For this review, take the finished solid that the model builds, in its own axes (mm). A direction names the side the tool comes from. Round coordinates to 2 decimals unless told otherwise and drop trailing zeros. Write each loop counter-clockwise with the first axis right and the second up, starting at its lowest first coordinate (ties: lowest second). Pieces come first, ordered by that corner, then holes. Notation, with made-up numbers: (-24, 80) -> (18, 80) arc R27 cw to (18, 107) -> close; hole circle Ø4 at (-31, -36.75). An arc over 180 degrees is marked (long way). Answer as CSV lines item,"result". Start each with the question number.
Item 1: Take a section at C-C on x = -47. Give the boundary of the cut face in (y, z).
Item 2: Take a section at D-D on x = 3. Give the boundary of the cut face in (y, z), then the cut area to 3 significant figures.
Item 3: Machinability: for faces 4 (the flat face through (-14, -12, 4)), 5 (the flat face through (0, 0, 8)), which of the approach directions +Z, -Z, +X, -X, +Y, -Y give a long, thin tool a straight path to every point of the face, cutting with its end or side? Answer none if there is none.
Item 4: Mouldability with a two-part tool opening along Y and no side actions: class faces 1 (the cylindrical face through (24.4, -44.6, 2)), 2 (the cylindrical face through (-13.887, -10.648, 5.972)), 3 (the flat face through (-1, 1, 0)) as +Y half, -Y half, draft (parallel to the pull), parting line (faces both ways), or undercut.
Item 5: For pin 1 Ø1.5 at (y, z) = (-25.5, 1) entering from +X; pin 2 Ø10 at (x, y) = (-43.5, -30.5) entering from +Z; pin 3 Ø5 at (x, y) = (23.5, -40.7) entering from +Z; pin 4 Ø6 at (x, y) = (-20.5, -11) entering from -Z, all flat-tipped, find the tip position at first contact; note any pin that passes through.
Item 6: Take a section at B-B on x = 23.5. Give the boundary of the cut face in (y, z).
Item 7: Take a section at A-A on y = 0. Give the boundary of the cut face in (x, z).
Item 8: Wall thickness on probe 1 along Y at (x, z) = (23.5, 3.05); probe 2 along Z at (x, y) = (-24.5, -42.5); probe 3 along X at (y, z) = (-40, 2.5): over which ranges is each line inside the solid? List them lowest first. Write a range as from..to.
```python
from build123d import *

# Parameters (mm, degrees)
SKETCH_1_R               = 57.5
EXTRUDE_1_DEPTH          = 4
SKETCH_2_R               = 17.5
EXTRUDE_2_DEPTH          = 4
SKETCH_3_R               = 4
CUT_EXTRUDE_1_DEPTH      = 12
PATTERN_CIRCULAR_1_COUNT = 3


with BuildPart() as part:
    # 草图1 → 凸台-拉伸1 (new body)
    with BuildSketch(Plane.XY):
        Circle(SKETCH_1_R)
    extrude(amount=EXTRUDE_1_DEPTH)

    # 草图2 → 凸台-拉伸2 (add)
    with BuildSketch(Plane.XY.offset(4)):
        Circle(SKETCH_2_R)
    extrude(amount=EXTRUDE_2_DEPTH)

    # 草图3 → 切除-拉伸1 (cut)
    with BuildSketch(Plane(origin=(0, 0, 0), x_dir=(-1, 0, 0), z_dir=(0, 0, -1))):
        with Locations((47, 0)):
            Circle(SKETCH_3_R)
    cut_extrude_1 = extrude(amount=-CUT_EXTRUDE_1_DEPTH, mode=Mode.SUBTRACT)

    # 阵列(圆周)1: 切除-拉伸1 ×3 about axis
    pattern_circular_1_axis = Axis((0, 0, 0), (0, 0, 1))
    for i in range(1, PATTERN_CIRCULAR_1_COUNT):
        add(cut_extrude_1.rotate(pattern_circular_1_axis, i * 360 / PATTERN_CIRCULAR_1_COUNT), mode=Mode.SUBTRACT)


solid = part.part
```
Output values:
1,outline,"(-33.12, 0) -> (-4, 0) -> (-4, 4) -> (-33.12, 4) -> close; (4, 0) -> (33.12, 0) -> (33.12, 4) -> (4, 4) -> close"
2,outline,"(-57.42, 0) -> (57.42, 0) -> (57.42, 4) -> (17.24, 4) -> (17.24, 8) -> (-17.24, 8) -> (-17.24, 4) -> (-57.42, 4) -> close"
2,area,"597 mm^2"
3,face 4,"+Z"
3,face 5,"+Z, +X, -X, +Y, -Y"
4,face 1,"undercut"
4,face 2,"parting line"
4,face 3,"draft"
5,pin 1,"stops at x = 51.9"
5,pin 2,"stops at z = 4"
5,pin 3,"passes through"
5,pin 4,"stops at z = 0"
6,outline,"(-52.48, 0) -> (-44.7, 0) -> (-44.7, 4) -> (-52.48, 4) -> close; (-36.7, 0) -> (36.7, 0) -> (36.7, 4) -> (-36.7, 4) -> close; (44.7, 0) -> (52.48, 0) -> (52.48, 4) -> (44.7, 4) -> close"
7,outline,"(-57.5, 0) -> (-51, 0) -> (-51, 4) -> (-57.5, 4) -> close; (-43, 0) -> (57.5, 0) -> (57.5, 4) -> (17.5, 4) -> (17.5, 8) -> (-17.5, 8) -> (-17.5, 4) -> (-43, 4) -> close"
8,probe 1,"y = -52.48..-44.7, -36.7..36.7, 44.7..52.48"
8,probe 2,"z = 0..4"
8,probe 3,"x = -41.31..19.56, 27.44..41.31"
